Autodesk Inventor part; units mm, degrees
ref_plane "YZ Plane" through (0, 0, 0) normal (1, 0, 0) x (0, 1, 0)
ref_plane "XZ Plane" through (0, 0, 0) normal (0, 1, 0) x (-1, 0, 0)
ref_plane "XY Plane" through (0, 0, 0) normal (0, 0, 1) x (1, 0, 0)
sketch "Sketch1" plane through (0, 0, 0) normal (0, 1, 0) x (-1, 0, 0)
  line L0 (-25, 25) -> (25, 25)
  line L1 (25, 25) -> (25, -25)
  line L2 (25, -25) -> (-25, -25)
  line L3 (-25, -25) -> (-25, 25)
  line L4 (-25, 25) -> (25, -25) construction
  line L5 (25, 25) -> (-25, -25) construction
  point P0 (0, 0)
  dimension "d0" = 50
  dimension "d1" = 50
extrude "Extrusion1" add sketch "Sketch1" along normal blind 36.5
sketch "Sketch2" plane through (-25, 0, 25) normal (0, 0, 1) x (1, 0, 0)
  line L0 (0, 0) -> (50, 0)
  line L1 (50, 0) -> (50, 36.5)
  line L2 (0, 36.5) -> (50, 36.5)
  line L3 (0, 0) -> (0, 36.5)
  circle A0 centre (40.7, 23.5) radius 6
  line L4 (25, 0) -> (25, 36.5) construction
  dimension "d4" = 15.7
  dimension "d5" = 13
  dimension "d6" = 12
extrude "Extrusion2" add sketch "Sketch2" along normal blind 19 contours A0
sketch "Sketch3" plane through (15.7, 23.5, 44) normal (0, 0, 1) x (1, 0, 0)
  circle A0 centre (0, 0) radius 6
  circle A1 centre (0, 0) radius 5
  point P0 (-15.7, -23.5)
  dimension "d9" = 10
extrude "Extrusion3" add sketch "Sketch3" along normal blind 26 contours A1
sketch "Sketch4" plane through (0, 36.5, 0) normal (0, 1, 0) x (1, 0, 0)
  circle A0 centre (0, 0) radius 19.25
  dimension "d12" = 38.5
extrude "Extrusion4" add sketch "Sketch4" along normal blind 35
sketch "Sketch5" plane through (15.7, 23.5, 70) normal (0, 0, 1) x (1, 0, 0)
  circle A0 centre (0, 0) radius 5
  circle A1 centre (0, 0) radius 4.5
  point P0 (-15.7, -23.5)
  dimension "d15" = 9
extrude "Extrusion5" cut sketch "Sketch5" against normal blind 12
sketch "Sketch6" plane through (0, 0, 0) normal (1, 0, 0) x (0, 1, 0)
  line L0 (28, 58) -> (19, 58)
  line L1 (28, 70) -> (19, 70)
  circle A0 centre (23.5, 65) radius 2.5
  point P0 (0, 0)
  point P1 (23.5, 70)
  dimension "d18" = 5
  dimension "d19" = 5
extrude "Extrusion6" cut sketch "Sketch6" along normal through all
sketch "Sketch7" plane through (25, 0, -25) normal (0, 0, -1) x (-1, 0, 0)
  line L0 (0, 0) -> (50, 0)
  line L1 (50, 0) -> (50, 36.5)
  line L2 (0, 36.5) -> (50, 36.5)
  line L3 (0, 0) -> (0, 36.5)
  line L4 (12.5, 22.5) -> (37.5, 22.5) construction
  point P0 (25, 0)
  point P1 (25, 22.5)
  point P2 (25, 0)
  dimension "d22" = 25
  dimension "d23" = 22.5
sketch "Sketch8" plane through (15.7, 23.5, 70) normal (0, 0, 1) x (1, 0, 0)
  circle A0 centre (0, 0) radius 4.5
  point P0 (-15.7, -23.5)
hole "Hole1" at (15.7, 23.5, 70) direction (0, 0, -1) diameter 5 depth 8
hole "Hole2" at (12.5, 22.5, -25) at (-12.5, 22.5, -25) direction (0, 0, 1) diameter 4.134 depth 8
sketch "Sketch9" plane through (-25, 0, -25) normal (-1, 0, 0) x (0, 0, 1)
  line L0 (0, 0) -> (50, 0)
  line L1 (50, 0) -> (50, 36.5)
  line L2 (0, 36.5) -> (50, 36.5)
  line L3 (0, 0) -> (0, 36.5)
  line L4 (12.5, 22.5) -> (37.5, 22.5) construction
  point P0 (25, 0)
  point P1 (25, 22.5)
  point P2 (25, 0)
  dimension "d38" = 25
  dimension "d39" = 22.5
hole "Hole3" at (-25, 22.5, -12.5) at (-25, 22.5, 12.5) direction (1, 0, 0) diameter 4.134 depth 8
chamfer "Chamfer1" distance 0.5 angle 45 4 edges at (25, 18.25, 25) (-25, 18.25, 25) (25, 18.25, -25) (-25, 18.25, -25)
properties part number "RE38S-600Z-1M" material "ABS Plastic"
For this review, take the finished solid that the model builds, in its own axes (mm). A direction names the side the tool comes from. Give positions to 0.01 mm unless a question says otherwise; leave off trailing zeros. Loops run counter-clockwise (first coordinate to the right, second up) from the corner with the lowest first, then second, coordinate; pieces in that order, holes last. Notation, with made-up numbers: M 14.25,85.25 L 73.25,85.25 A20 ccw 73.25,96.25 Z; hole C 53.25,77 d7. An arc over 180 degrees is marked long. One line per item, written item: value. Start each with the question number.
Q1. For L1, parallel to X at y = 22.5, z = -20; L2, parallel to Z at x = 14.75, y = 23.5, list the stretches that pass through material, from the lowest coordinate up.
Q2. Draft analysis for pull direction Y (two halves, no side actions). For faces 1 (the face through (0, 0, 0)), 2 (the face through (11, 24, 58)), 3 (the face through (-11.71, 24.41, -20.94)), state which applies: released by +Y, released by -Y, zero draft, split by the parting line, or undercut.
Q3. Clearance check with flat-ended pins moving along their axes: pin 1 Ø18 at (x, y) = (4.5, 15.5) entering from +Z; pin 2 Ø3 at (x, z) = (10, 35.5) entering from +Y; pin 3 Ø8 at (y, z) = (57, -12.5) entering from +X. State where each tip first meets the part, or that it passes through.
Q4. Machinability: for faces 4 (the face through (13, 28, 44)), 5 (the face through (18, 21, 65)), 6 (the face through (-17, 22, -13)), 7 (the face through (-15.28, 53.76, -11.71)), 8 (the face through (-13, 22, -17)), which of the approach directions +Z, -Z, +X, -X, +Y, -Y give a long, thin tool a straight path to every point of the face, cutting with its end or side? Answer none if there is none.
Q5. Add section C-C (z = 39). Give the boundary of the cut face in (x, y), and give its area (3 significant figures).
Q6. Add section A-A (y = 11.5). Give the boundary of the cut face in (x, z), and give its area (3 significant figures).
Q7. Add section B-B (x = -3.5). Give the boundary of the cut face in (y, z), and give its area (3 significant figures).
Q8. Add section D-D (z = -12.5). Give the boundary of the cut face in (x, y), and give its area (3 significant figures).
Reply:
1. L1: -25 to -14.57, -10.43 to 10.43, 14.57 to 25
1. L2: -25 to 62
2. face 1: released by -Y
2. face 2: zero draft
2. face 3: undercut
3. pin 1: z = 58
3. pin 2: y = 27.78
3. pin 3: x = 17.27
4. face 4: +Z
4. face 5: +X, -X
4. face 6: -X
4. face 7: +Y
4. face 8: -Z
5. outline: C 15.7,23.5 d12
5. area: 113 mm²
6. outline: M -25,-24.5 L -24.5,-25 L 24.5,-25 L 25,-24.5 L 25,24.5 L 24.5,25 L -24.5,25 L -25,24.5 Z
6. area: 2,500 mm²
7. outline: M 0,-25 L 36.5,-25 L 36.5,-18.93 L 71.5,-18.93 L 71.5,18.93 L 36.5,18.93 L 36.5,25 L 0,25 Z
7. area: 3,150 mm²
8. outline: M -25,0 L 25,0 L 25,36.5 L 14.64,36.5 L 14.64,71.5 L -14.64,71.5 L -14.64,36.5 L -25,36.5 L -25,24.57 L -17,24.57 L -17,20.43 L -25,20.43 Z
8. area: 2,820 mm²
